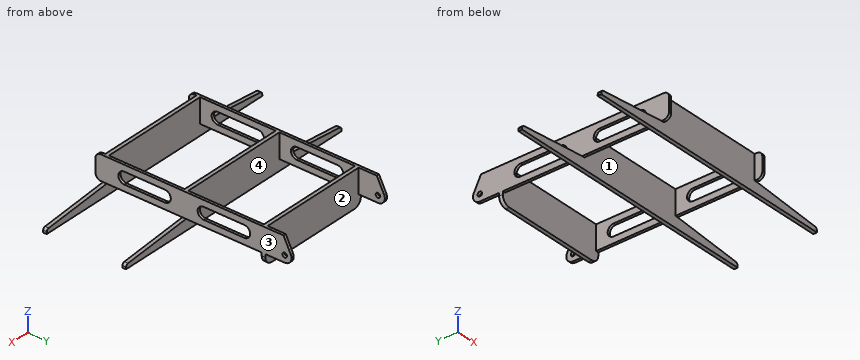
```python
from build123d import *

# Parameters (mm, degrees)
SKETCH1_W               = 1237.47
SKETCH1_H               = 14
BOSS_EXTRUDE1_DEPTH     = 133
LPATTERN1_COUNT         = 3
LPATTERN1_PITCH         = 300
CUT_EXTRUDE1_DEPTH      = 882.76981136
CUT_EXTRUDE1_DEPTH_BACK = 882.76981136
SKETCH3_W               = 91.96189972
SKETCH3_H               = 741.26
BOSS_EXTRUDE2_DEPTH     = 10
SKETCH4_W               = 289.906679044
SKETCH4_H               = 376.133897458
CUT_EXTRUDE3_DEPTH      = 105
CUT_EXTRUDE5_DEPTH      = 960.881700163
CUT_EXTRUDE5_DEPTH_BACK = 960.881700163
SKETCH5_R               = 8.65
FILLET1_R               = 30
FILLET2_R               = 20
FILLET3_R               = 10
CUT_EXTRUDE6_DEPTH      = 960.881700163
CUT_EXTRUDE6_DEPTH_BACK = 960.881700163


with BuildPart() as part:
    # Sketch1 → Boss-Extrude1 (new body)
    with BuildSketch(Plane.XY):
        Rectangle(SKETCH1_W, SKETCH1_H)
    extrude(amount=BOSS_EXTRUDE1_DEPTH)


with BuildPart() as lpattern1_1:
    # LPattern1: pattern copy
    add(part.part.moved(Location(Vector(0, -1, 0) * (1 * LPATTERN1_PITCH))))


with BuildPart() as lpattern1_2:
    # LPattern1: pattern copy
    add(part.part.moved(Location(Vector(0, -1, 0) * (2 * LPATTERN1_PITCH))))


with BuildPart() as cut_extrude1_tool:
    # Sketch2 → Cut-Extrude1 (new, two sides: drawn at the far end of the back side and taken through both)
    with BuildSketch(Plane(origin=(0, 7, 0), x_dir=(1, 0, 0), z_dir=(0, 1, 0)).offset(-CUT_EXTRUDE1_DEPTH_BACK)):
        Polygon((-675.17481683, 0), (-675.17481683, -133), (-217.007056567, -133), (-217.007056567, -41.03810028), (-488.641898603, -15.743660333), (-489.975, 0), align=None)
        Polygon((489.975, 0), (675.17481683, 0), (675.17481683, -133), (217.007056567, -133), (217.007056567, -41.03810028), (488.641898603, -15.743660333), align=None)
    extrude(amount=CUT_EXTRUDE1_DEPTH + CUT_EXTRUDE1_DEPTH_BACK)


with BuildPart() as part_1:
    add(part.part)

    # Cut-Extrude1: cut by cut_extrude1_tool
    add(cut_extrude1_tool.part, mode=Mode.SUBTRACT)



with BuildPart() as lpattern1_1_1:
    add(lpattern1_1.part)

    # Cut-Extrude1: cut by cut_extrude1_tool
    add(cut_extrude1_tool.part, mode=Mode.SUBTRACT)


with BuildPart() as lpattern1_2_1:
    add(lpattern1_2.part)

    # Cut-Extrude1: cut by cut_extrude1_tool
    add(cut_extrude1_tool.part, mode=Mode.SUBTRACT)


with BuildPart() as part_2:
    add(part_1.part)

    add(lpattern1_1_1.part)  # Boss-Extrude2 merges LPattern1_1

    add(lpattern1_2_1.part)  # Boss-Extrude2 merges LPattern1_2
    # Sketch3 → Boss-Extrude2 (add)
    with BuildSketch(Plane.ZY.offset(217.007056567)):
        with Locations((87.01905014, -264.87)):
            Rectangle(SKETCH3_W, SKETCH3_H)
    boss_extrude2 = extrude(amount=-BOSS_EXTRUDE2_DEPTH)

    # Mirror1: Boss-Extrude2 across plane
    add(boss_extrude2.mirror(Plane(origin=(0, 0, 0), x_dir=(0, 0, 1), z_dir=(1, 0, 0))))

    # Sketch4 → Cut-Extrude3 (cut)
    with BuildSketch(Plane(origin=(0, 7, 0), x_dir=(1, 0, 0), z_dir=(0, 1, 0))):
        with Locations((-361.960396089, -44.135281773)):
            Rectangle(SKETCH4_W, SKETCH4_H)
        with Locations((361.960396089, -44.135281773)):
            Rectangle(SKETCH4_W, SKETCH4_H)
    extrude(amount=-CUT_EXTRUDE3_DEPTH, mode=Mode.SUBTRACT)

    # Sketch5 → Cut-Extrude5 (cut, two sides: drawn at the far end of the back side and taken through both)
    with BuildSketch(Plane(origin=(217.007056567, 0, 0), x_dir=(0, 0, -1), z_dir=(1, 0, 0)).offset(-CUT_EXTRUDE5_DEPTH_BACK)):
        with BuildLine():
            Line((-133, 105.76), (-133, 75.48))
            Line((-133, 75.48), (-78.550242405, 102.979525411))
            ThreePointArc((-78.550242405, 102.979525411), (-53.345094409, 101.921723933), (-41.03810028, 79.9))
            Line((-41.03810028, 79.9), (-41.03810028, 105.76))
            Line((-41.03810028, 105.76), (-133, 105.76))
        make_face()
        with Locations(Location((-66.89810028, 79.9, 0), (0, 0, 90))):
            Circle(SKETCH5_R)
    extrude(amount=CUT_EXTRUDE5_DEPTH + CUT_EXTRUDE5_DEPTH_BACK, mode=Mode.SUBTRACT)

    # Fillet1
    fillet1_edges = [part_2.edges().sort_by_distance(p)[0] for p in [
        (-217.007056567, 0, 0),
        (217.007056567, 0, 0),
    ]]
    fillet(fillet1_edges, radius=FILLET1_R)

    # Fillet2
    fillet2_edges = [part_2.edges().sort_by_distance(p)[0] for p in [
        (212.007056567, -635.5, 133),
        (212.007056567, -635.5, 41.03810028),
        (-212.007056567, -635.5, 41.03810028),
        (-212.007056567, -635.5, 133),
    ]]
    fillet(fillet2_edges, radius=FILLET2_R)

    # Fillet3
    fillet3_edges = [part_2.edges().sort_by_distance(p)[0] for p in [
        (488.641898603, -300, 15.743660333),
        (-488.641898603, -300, 15.743660333),
        (488.641898603, -600, 15.743660333),
        (-488.641898603, -600, 15.743660333),
    ]]
    fillet(fillet3_edges, radius=FILLET3_R)

    # Sketch6 → Cut-Extrude6 (cut, two sides: drawn at the far end of the back side and taken through both)
    with BuildSketch(Plane.ZY.offset(217.007056567).offset(-CUT_EXTRUDE6_DEPTH_BACK)):
        with BuildLine():
            Line((109.24905014, -73.05), (109.24905014, -226.95))
            ThreePointArc((109.24905014, -226.95), (87.01905014, -249.18), (64.78905014, -226.95))
            Line((64.78905014, -226.95), (64.78905014, -73.05))
            ThreePointArc((64.78905014, -73.05), (87.01905014, -50.82), (109.24905014, -73.05))
        make_face()
        with BuildLine():
            Line((109.24905014, -373.05), (109.24905014, -526.95))
            ThreePointArc((109.24905014, -526.95), (87.01905014, -549.18), (64.78905014, -526.95))
            Line((64.78905014, -526.95), (64.78905014, -373.05))
            ThreePointArc((64.78905014, -373.05), (87.01905014, -350.82), (109.24905014, -373.05))
        make_face()
    extrude(amount=CUT_EXTRUDE6_DEPTH + CUT_EXTRUDE6_DEPTH_BACK, mode=Mode.SUBTRACT)


solid = part_2.part
```
Can you work these out from the model? Positions are in its coordinate system, mm. Face numbers are marked on the shaded views. Give positions to 0.01 mm unless a question says otherwise; leave off trailing zeros. Write each loop counter-clockwise with the first axis right and the second up, starting at its lowest first coordinate (ties: lowest second). Pieces come first, ordered by that corner, then holes. Notation, with made-up numbers: (-35.5, 48.5) - (-20.5, 48.5) arc R10 ccw to (-20.5, 60.5) - close; hole circle Ø8 at (30, 0). An arc over 180 degrees is marked (long way). Write item = value, one per line. Start each with the question number.
1. Imagine slicing it at C-C (x = -420). Please give me the cut outline in (y, z), and give its area (3 significant figures).
2. For pin 1 (3 mm diameter, centred on x = -214.5, y = -125.5, fed in from -Z); pin 2 (12 mm diameter, centred on y = -31, z = 115, fed in from +X); pin 3 (6 mm diameter, centred on x = 159, z = 37.5, fed in from +Y), each with a flat end and sliding along its axis, tell me the tip position at first contact or that it passes through.
3. Imagine slicing it at A-A (y = -392). Please give me the cut outline in (x, z), and give its area (3 significant figures).
4. Imagine slicing it at B-B (x = 293). Please give me the cut outline in (y, z).
5. Thinking about a two-plate mould opening in Y: for the marked faces 1, 2, 3 and 4, which applies, released by +Y, released by -Y, zero draft, split by the parting line, or undercut?
6. Please list where these lines run through material, in increasing order: line 1 (Y direction, x = 133, z = 49); line 2 (X direction, y = -324, z = 68.5); line 3 (Z direction, x = 210, y = 79).
Worked answers:
q1.outline = (-607, 0) - (-593, 0) - (-593, 22.14) - (-607, 22.14) - close; (-307, 0) - (-293, 0) - (-293, 22.14) - (-307, 22.14) - close
q1.area = 620 mm2
q2.pin_1 = 41.04
q2.pin_2 = 217.01
q2.pin_3 = 7
q3.outline = (-217.01, 41.04) - (-207.01, 41.04) - (-207.01, 64.79) - (-217.01, 64.79) - close; (-217.01, 109.25) - (-207.01, 109.25) - (-207.01, 133) - (-217.01, 133) - close; (207.01, 41.04) - (217.01, 41.04) - (217.01, 64.79) - (207.01, 64.79) - close; (207.01, 109.25) - (217.01, 109.25) - (217.01, 133) - (207.01, 133) - close
q3.area = 950 mm2
q4.outline = (-607, 0) - (-593, 0) - (-593, 33.96) - (-607, 33.96) - close; (-307, 0) - (-293, 0) - (-293, 33.96) - (-307, 33.96) - close
q5.face_1 = undercut
q5.face_2 = released by +Y
q5.face_3 = zero draft
q5.face_4 = undercut
q6.line_1 = -607 to -593, -307 to -293, -7 to 7
q6.line_2 = -217.01 to -207.01, 207.01 to 217.01
q6.line_3 = 41.04 to 58.3, 75.5 to 126.03
